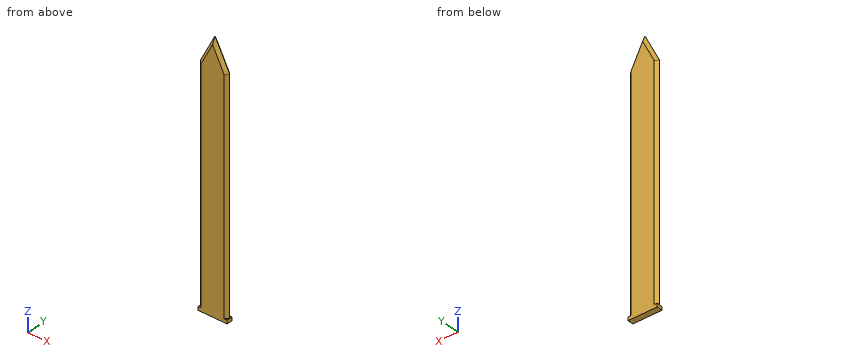
from build123d import *

# Parameters (mm, degrees)
F0_W     = 76.2
F0_H     = 304.8
F1_DEPTH = 7.62
F2_SIZE  = 7.61999
F3_W     = 76.2
F3_H     = 9.4219583702
F4_DEPTH = 15.24


# Not quite as in the source:
# - a fillet or chamfer is up to 0.001 mm smaller than in the source, because OpenCascade refuses the exact size


with BuildPart() as f1:
    # F0 (on Front) → F1 (new body, symmetric)
    with BuildSketch(Plane.XZ):
        with Locations((0, -152.4)):
            Rectangle(F0_W, F0_H)
        with Locations((0, 152.4)):
            Rectangle(F0_W, F0_H)
        Polygon((-38.1, 304.8), (38.1, 304.8), (0, 381), align=None)
    extrude(amount=F1_DEPTH, both=True)

    # F2 (size 7.62 in the source; OpenCascade refuses exactly that, so slightly less here)
    f2_edges = [f1.edges().sort_by_distance(p)[0] for p in [
        (0, -7.62, -304.8),
        (38.1, -7.62, 0),
        (19.05, -7.62, 342.9),
        (-19.05, -7.62, 342.9),
        (-38.1, -7.62, 0),
        (0, 7.62, -304.8),
        (38.1, 7.62, 0),
        (19.05, 7.62, 342.9),
        (-19.05, 7.62, 342.9),
        (-38.1, 7.62, 0),
    ]]
    chamfer(f2_edges, length=F2_SIZE)

    # F3 (on face) → F4 (join)
    with BuildSketch(Plane.XZ.offset(7.62)):
        with Locations((0, -301.8909791851)):
            Rectangle(F3_W, F3_H)
    extrude(amount=-F4_DEPTH)


solid = f1.part
Build history of the part. All positions in model axes, mm. Coordinates: 2 decimals unless noted, no trailing zeros. Order: outer loops, then holes, each group sorted by start corner. A loop starts at its lowest first (then second) coordinate and runs counter-clockwise, first axis right, second up. Notation, with made-up numbers: (29, -3.75) - (73, -3.75) arc R15 ccw to (73, 2.25) - close; hole circle Ø1 at (15, -31). An arc over 180 degrees is marked (long way). Put each result on its own line as item: value.
1. Saw through at C-C (y = 3). Write the cut outline in (x, z).
Answer sheet:
outline: (-38.1, -306.6) - (38.1, -306.6) - (38.1, -297.18) - (35.1, -297.18) - (35.1, 304.09) - (0, 374.29) - (-35.1, 304.09) - (-35.1, -297.18) - (-38.1, -297.18) - close
2. Drop flat-ended pins along their axis: P1, Ø6, axis at y = -4.5, z = -149, coming from the -X side; P2, Ø2, axis at y = 3, z = 83.5, coming from the +X side; P3, Ø1, axis at y = -5, z = 304, coming from the -X side. Give the stop position or say it passes through.
Answer sheet:
P1: stops at x = -36.6
P2: stops at x = 36.1
P3: stops at x = -33.52
3. Probe line 1 along Z through (x, y) = (-4, 0.25); line 2 along X through (y, z) = (-2.75, -106); line 3 along Z through (x, y) = (-32, 5.5). List the from-to ranges inside material, lowest first. Write a range as [from, to].
Answer sheet:
line 1: z = [-306.6, 372.44]
line 2: x = [-35.35, 35.35]
line 3: z = [-306.6, 304.7]
